Could you check a few things on this model? Use its own coordinates, in mm. Face numbers are marked on the shaded views. A direction names the side the tool comes from. Give positions to 0.01 mm unless a question says otherwise; leave off trailing zeros. Loops run counter-clockwise (first coordinate to the right, second up) from the corner with the lowest first, then second, coordinate; pieces in that order, holes last. Notation, with made-up numbers: M -31.75,-35.75 L -3.75,-35.75 A15 cw -3.75,-14.75 Z; hole C 73.5,79 d8. An arc over 180 degrees is marked long. Answer in a Markdown table with one row per item. Add a question column.
```python
from build123d import *

# Parameters (mm, degrees)
SKETCH_1_W      = 15
SKETCH_1_H      = 7
SKETCH_1_W_2    = 4.5
SKETCH_1_H_2    = 3.3
EXTRUDE_1_DEPTH = 0.4
SKETCH_2_W      = 15
SKETCH_2_H      = 7
EXTRUDE_2_DEPTH = 6.6
SKETCH_3_W      = 8.6
SKETCH_3_H      = 7
EXTRUDE_3_DEPTH = 0.4
SKETCH_4_W      = 8.6
SKETCH_4_H      = 7
EXTRUDE_4_DEPTH = 0.4
SKETCH_5_W      = 2.417347104
SKETCH_5_H      = 2.320372832
EXTRUDE_5_DEPTH = 6.1


with BuildPart() as part:
    # Эскиз1 → Бобышка-Вытянуть1 (new body)
    with BuildSketch(Plane.XY):
        with Locations((7.5, 3.5)):
            Rectangle(SKETCH_1_W, SKETCH_1_H)
        with Locations((7.5, 3.5)):
            Rectangle(SKETCH_1_W_2, SKETCH_1_H_2, mode=Mode.SUBTRACT)
    extrude(amount=EXTRUDE_1_DEPTH)

    # Эскиз2 → Бобышка-Вытянуть2 (add)
    with BuildSketch(Plane(origin=(0, 0, 0), x_dir=(-1, 0, 0), z_dir=(0, 0, -1))):
        with Locations((-7.5, 3.5)):
            Rectangle(SKETCH_2_W, SKETCH_2_H)
    extrude(amount=EXTRUDE_2_DEPTH)

    # Эскиз3 → Бобышка-Вытянуть3 (add)
    with BuildSketch(Plane(origin=(15, 0, 0), x_dir=(0, 0, -1), z_dir=(1, 0, 0))):
        with Locations((3.9, 3.5)):
            Rectangle(SKETCH_3_W, SKETCH_3_H)
    extrude(amount=-EXTRUDE_3_DEPTH)

    # Эскиз4 → Бобышка-Вытянуть4 (add)
    with BuildSketch(Plane.ZY):
        with Locations((-3.9, 3.5)):
            Rectangle(SKETCH_4_W, SKETCH_4_H)
    extrude(amount=-EXTRUDE_4_DEPTH)

    # Эскиз5 → Бобышка-Вытянуть5 (add)
    with BuildSketch(Plane.XY):
        with Locations((6.472493098, 3.5)):
            Rectangle(SKETCH_5_W, SKETCH_5_H)
    extrude(amount=EXTRUDE_5_DEPTH)


solid = part.part
```
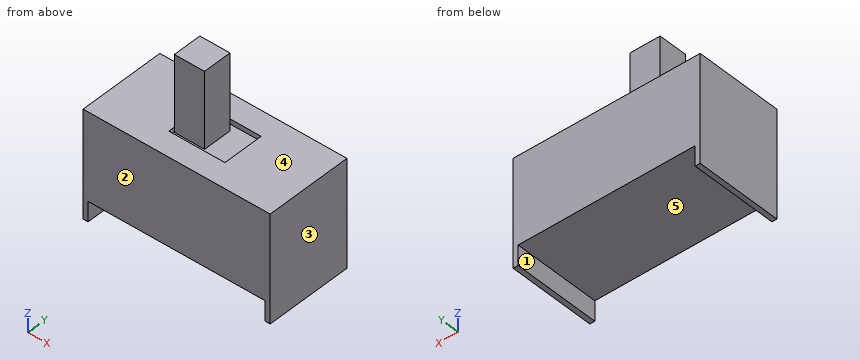
Item 1: I need wall thicknesses on L1, parallel to Z at x = 8, y = 1.5; L2, parallel to X at y = 3, z = 0.5; L3, parallel to Z at x = 6.5, y = 3. Which ranges of each line are inside material? Lowest first, please.
Item 2: Suppose I cut it at B-B (y = 5.5). List the corners of the cut face in (x, z) for me.
Item 3: If we mould it in two halves opening along X, with no side actions, what happens to the marked faces 3, 4 and 5? For each: +X half, -X half, draft (parallel to the pull), parting line (faces both ways), or undercut.
Item 4: Suppose I cut it at A-A (x = 9.25). List the corners of the cut face in (y, z) for me, then the cut area to 3 significant figures.
Item 5: Suppose I cut it at C-C (z = 5). List the corners of the cut face in (x, y) for me.
Item 6: Suppose I cut it at D-D (x = 6.5). List the corners of the cut face in (y, z) for me.
Item 7: For the marked faces 1 and 2, which set-ups out of +Z, -Z, +X, -X, +Y, -Y let a thin tool reach every point of the face, with its end or its side?
Item 8: For P1, Ø2, axis at x = 4.5, y = 5, coming from the -Z side; P2, Ø1, axis at x = 6, y = 6, coming from the +Z side; P3, Ø1.2, axis at y = 3.5, z = 2.5, coming from the -X side, each with a flat end and sliding along its axis, tell me the tip position at first contact or that it passes through.
Values found:
| question | item | result |
|---|---|---|
| 1 | L1 | -6.6 to 0.4 |
| 1 | L2 | 5.26 to 7.68 |
| 1 | L3 | -6.6 to 6.1 |
| 2 | outline | M 0,-8.2 L 0.4,-8.2 L 0.4,-6.6 L 14.6,-6.6 L 14.6,-8.2 L 15,-8.2 L 15,0.4 L 0,0.4 Z |
| 3 | face 3 | +X half |
| 3 | face 4 | draft |
| 3 | face 5 | undercut |
| 4 | outline | M 0,-6.6 L 7,-6.6 L 7,0.4 L 5.15,0.4 L 5.15,0 L 1.85,0 L 1.85,0.4 L 0,0.4 Z |
| 4 | area | 47.7 mm² |
| 5 | outline | M 5.26,2.34 L 7.68,2.34 L 7.68,4.66 L 5.26,4.66 Z |
| 6 | outline | M 0,-6.6 L 7,-6.6 L 7,0.4 L 5.15,0.4 L 5.15,0 L 4.66,0 L 4.66,6.1 L 2.34,6.1 L 2.34,0 L 1.85,0 L 1.85,0.4 L 0,0.4 Z |
| 7 | face 1 | -Z, +Y, -Y |
| 7 | face 2 | +Z, -Z, +X, -X, -Y |
| 8 | P1 | z = -6.6 |
| 8 | P2 | z = 0.4 |
| 8 | P3 | x = 5.26 |
